from build123d import *

# Parameters (mm, degrees)
F0_R     = 8
F0_R_2   = 6
F0_R_3   = 5
F1_DEPTH = 235
F2_DEPTH = 40
F3_R     = 5
F4_DEPTH = 15
F5_R     = 5
F6_DEPTH = 10


with BuildPart() as f1:
    # F0 (on Front) → F1 (new body)
    with BuildSketch(Plane.XZ):
        with Locations((-6.1693550088, 11.2500013784)):
            Circle(F0_R)
        with Locations((-6.1693550088, 11.2500013784)):
            Circle(F0_R_2, mode=Mode.SUBTRACT)
        with Locations((-6.1693550088, 11.2500013784)):
            Circle(F0_R_2)
        with Locations((-6.1693550088, 11.2500013784)):
            Circle(F0_R_3, mode=Mode.SUBTRACT)
        with Locations((-6.1693550088, 11.2500013784)):
            Circle(F0_R_3)
    extrude(amount=F1_DEPTH)

    # F0 (on Front) → F2 (join)
    with BuildSketch(Plane.XZ):
        with Locations((-6.1693550088, 11.2500013784)):
            Circle(F0_R_2)
        with Locations((-6.1693550088, 11.2500013784)):
            Circle(F0_R_3, mode=Mode.SUBTRACT)
        with Locations((-6.1693550088, 11.2500013784)):
            Circle(F0_R_3)
    extrude(amount=-F2_DEPTH)

    # F3 (on face) → F4 (join)
    with BuildSketch(Plane(origin=(0, 40, 0), x_dir=(-1, 0, 0), z_dir=(0, 1, 0))):
        with Locations((6.1693550088, 11.2500013784)):
            Circle(F3_R)
    extrude(amount=F4_DEPTH)

    # F5 (on face) → F6 (join)
    with BuildSketch(Plane.XZ.offset(235)):
        with Locations((-6.1693550088, 11.2500013784)):
            Circle(F5_R)
    extrude(amount=F6_DEPTH)


solid = f1.part
Part model, mm, in its own coordinate system. A direction names the side the tool comes from. Give positions to 0.01 mm unless a question says otherwise; leave off trailing zeros. Order: outer loops, then holes, each group sorted by start corner. A loop starts at its lowest first (then second) coordinate and runs counter-clockwise, first axis right, second up. Notation, with made-up numbers: (66, 21.5) - (120, 21.5) arc R19 ccw to (120, 51.5) - close; hole circle Ø3 at (-37, -29). An arc over 180 degrees is marked (long way). Use a Markdown table: item, result.
1) Probe L1, parallel to Y at x = -2.5, z = 15; L2, parallel to Y at x = -12, z = 7.75; L3, parallel to X at y = -81, z = 12. List the from-to ranges inside material, lowest first. Write a range as from..to.
Checked values:
| item | result |
|---|---|
| L1 | -235..40 |
| L2 | -235..0 |
| L3 | -14.13..1.8 |
2) Flat gauge pins, fed straight in: P1, Ø2, axis at y = -89, z = 13, coming from the +X side; P2, Ø1, axis at x = -5.5, y = -43, coming from the +Z side; P3, Ø4, axis at y = -49.5, z = 13.5, coming from the -X side. Where does each tip first touch, or does it go through?
Checked values:
| item | result |
|---|---|
| P1 | x = 1.8 |
| P2 | z = 19.25 |
| P3 | x = -14.17 |
3) Saw through at B-B on y = -204. List the corners of the cut face in (x, z).
Checked values:
| item | result |
|---|---|
| outline | circle Ø16 at (-6.17, 11.25) |
4) Saw through at C-C on y = 19. List the corners of the cut face in (x, z).
Checked values:
| item | result |
|---|---|
| outline | circle Ø12 at (-6.17, 11.25) |
5) Saw through at A-A on x = -5.25. List the corners of the cut face in (y, z), plus the area to 3 significant figures.
Checked values:
| item | result |
|---|---|
| outline | (-245, 6.34) - (-235, 6.34) - (-235, 3.3) - (0, 3.3) - (0, 5.32) - (40, 5.32) - (40, 6.34) - (55, 6.34) - (55, 16.16) - (40, 16.16) - (40, 17.18) - (0, 17.18) - (0, 19.2) - (-235, 19.2) - (-235, 16.16) - (-245, 16.16) - close |
| area | 4,460 mm² |
6) 3-axis set-ups, long thin cutter, end or side, ignore diameter. For faces 1 (the flat face through (-6, -245, 11)), 2 (the cylindrical face through (-6.82, -239.93, 16.207)), 3 (the cylindrical face through (-5.518, 47.395, 16.207)): which of +Z, -Z, +X, -X, +Y, -Y reach the whole face in a straight line?
Checked values:
| item | result |
|---|---|
| face 1 | +Z, -Z, +X, -X, -Y |
| face 2 | -Y |
| face 3 | +Y |
